from build123d import *

# Parameters (mm, degrees)
BOSS_EXTRUDE1_DEPTH      = 20
BOSS_EXTRUDE1_DEPTH_BACK = 20
SKETCH1_R                = 5
SKETCH1_R_2              = 6.5
CUT_EXTRUDE4_DEPTH       = 35
SKETCH6_R                = 1.5
CUT_EXTRUDE5_DEPTH       = 10
CUT_EXTRUDE6_DEPTH       = 50


with BuildPart() as part:
    # Sketch1 → Boss-Extrude1 (new, two sides: drawn at the far end of the back side and taken through both)
    with BuildSketch(Plane(origin=(0, 0, 0), x_dir=(1, 0, 0), z_dir=(0, 1, 0)).offset(-BOSS_EXTRUDE1_DEPTH_BACK)):
        with BuildLine():
            add(Edge.make_bspline(
                [(0, 20), (-114.873131821, 40.378289836), (-300, 56.568542495), (-328.284271247, 28.284271247)],
                knots=[0.1900067, 0.1900067, 0.1900067, 0.1900067, 1.1900067, 1.1900067, 1.1900067, 1.1900067], degree=3))
            ThreePointArc((-328.284271247, 28.284271247), (-328.284271247, -28.284271247), (-271.715728753, -28.284271247))
            add(Edge.make_bspline(
                [(-271.715728753, -28.284271247), (-194.91847241, 48.512985095), (-42.964488834, -10.495172733), (-6.202879594, -19.013791961)],
                knots=[0, 0, 0, 0, 0.930923327, 0.930923327, 0.930923327, 0.930923327], degree=3))
            ThreePointArc((-6.202879594, -19.013791961), (-1.015557257, -19.974199445), (4.242424242, -19.544867269))
            Line((4.242424242, -19.544867269), (35.757575758, -12.704163725))
            ThreePointArc((35.757575758, -12.704163725), (45.999746115, 0.081246157), (35.598568909, 12.737638699))
            Line((35.598568909, 12.737638699), (0, 20))
        make_face()
        with Locations(Location((0, 0, 0), (0, 0, 270))):
            Circle(SKETCH1_R, mode=Mode.SUBTRACT)
        with Locations(Location((33, 0, 0), (0, 0, 270))):
            Circle(SKETCH1_R_2, mode=Mode.SUBTRACT)
    extrude(amount=BOSS_EXTRUDE1_DEPTH + BOSS_EXTRUDE1_DEPTH_BACK)

    # Sketch5 → Cut-Extrude4 (cut)
    with BuildSketch(Plane(origin=(0, 20, 0), x_dir=(1, 0, 0), z_dir=(0, 1, 0))):
        Polygon((-47.037049996, 27.527548523), (92.120786702, 16.164640032), (85.724700256, -16.918764701), (-17.262768022, -30.907770073), align=None)
    extrude(amount=-CUT_EXTRUDE4_DEPTH, mode=Mode.SUBTRACT)

    # Sketch6 → Cut-Extrude5 (cut)
    with BuildSketch(Plane(origin=(0, -20, 0), x_dir=(-1, 0, 0), z_dir=(0, -1, 0))):
        with Locations(Location((23.950772589, -7.329216823, 0), (0, 0, 90))):
            Circle(SKETCH6_R)
        with Locations(Location((-16.971180087, -5.159042993, 0), (0, 0, 90))):
            Circle(SKETCH6_R)
        with Locations(Location((37.588692144, 19.43670737, 0), (0, 0, 90))):
            Circle(SKETCH6_R)
    extrude(amount=-CUT_EXTRUDE5_DEPTH, mode=Mode.SUBTRACT)

    # Sketch7 → Cut-Extrude6 (cut)
    with BuildSketch(Plane(origin=(0, 20, 0), x_dir=(1, 0, 0), z_dir=(0, 1, 0))):
        Polygon((-47.037049996, 27.527548523), (-26.137658318, -13.489817144), (-379.595719096, -92.580220424), (-321.505561991, 137.254748988), align=None)
    extrude(amount=-CUT_EXTRUDE6_DEPTH, mode=Mode.SUBTRACT)


solid = part.part
Geometry check sheet. Reference: the model listing, model coordinates, mm. Round coordinates to 2 decimals unless told otherwise and drop trailing zeros. Order: outer loops, then holes, each group sorted by start corner. A loop starts at its lowest first (then second) coordinate and runs counter-clockwise, first axis right, second up. Notation, with made-up numbers: (83, 54) - (92, 54) arc R17 ccw to (92, 84) - close; hole circle Ø11 at (19, 16.5). An arc over 180 degrees is marked (long way). One line per question, with ' | ' between items. Start each with the question number.
(1) Sectioned sample at C-C on y = -19.2. Count the separate pieces of the cut face and the enclosed holes in it, and give its area (3 significant figures).
(2) Sectioned sample at A-A on x = 31. Record the cut outline in (y, z), and give its area (3 significant figures).
(3) Sectioned sample at D-D on x = 13. Record the cut outline in (y, z), and give its area (3 significant figures).
(4) Depth check by flat-ended pin: pin 1 Ø2 at (x, y) = (27.5, -19) entering from +Z; pin 2 Ø2.5 at (x, z) = (-23.95, 7.33) entering from -Y; pin 3 Ø5 at (x, z) = (16.97, 5.16) entering from -Y; pin 4 Ø3 at (x, y) = (3, -17.5) entering from +Z. Enter the tip coordinate at first touch or a pass-through.
(5) Sectioned sample at B-B on z = -4. Record the cut outline in (x, y).
(6) Release check for a two-part mould opening along X. For faces 1 (the flat face through (-36.734, -17.465, -7.306)), 2 (the cylindrical face through (-4.88, -17.54, -1.08)), 3 (the cylindrical face through (-1.09, -17.54, 19.97)) record: released by +X, released by -X, zero draft, split by the parting line, or undercut.
(7) Thickness scan on L1, parallel to X at y = -19.2, z = 6; L2, parallel to X at y = -16.15, z = -4; L3, parallel to X at y = -18.9, z = 0. Record the ranges inside material, lowest first. Write a range as [from, to].
Conclusion:
1) separate pieces: 1 | enclosed holes: 5 | area: 2,560 mm2
2) outline: (-20, -13.68) - (-15, -13.68) - (-15, -6.18) - (-20, -6.18) - close; (-20, 6.18) - (-15, 6.18) - (-15, 13.74) - (-20, 13.74) - close | area: 75.2 mm2
3) outline: (-20, -17.35) - (-15, -17.35) - (-15, 17.64) - (-20, 17.64) - close | area: 175 mm2
4) pin 1: stops at z = 14.71 | pin 2: passes through | pin 3: stops at y = -20 | pin 4: stops at z = 19.94
5) outline: (-35.05, -20) - (-3, -20) - (-3, -15) - (-35.05, -15) - close; (3, -20) - (27.88, -20) - (27.88, -15) - (3, -15) - close; (38.12, -20) - (45.37, -20) - (45.37, -15) - (38.12, -15) - close
6) face 1: released by -X | face 2: undercut | face 3: split by the parting line
7) L1: x = [-29.95, -24.65], [-23.26, 15.73], [18.21, 30.5], [35.5, 44.53] | L2: x = [-35.05, -3], [3, 27.88], [38.12, 45.37] | L3: x = [-33.01, -5], [5, 26.5], [39.5, 46]
